For this review, take the finished solid that the model builds, in its own axes (mm). Face numbers are marked on the shaded views. A direction names the side the tool comes from. Coordinates: 2 decimals unless noted, no trailing zeros. Order: outer loops, then holes, each group sorted by start corner. A loop starts at its lowest first (then second) coordinate and runs counter-clockwise, first axis right, second up. Notation, with made-up numbers: (-14.5, 5.5) -> (-9.5, 5.5) arc R22 ccw to (-9.5, 24.5) -> close; hole circle Ø10 at (66.5, 53.5). An arc over 180 degrees is marked (long way). Return JSON: item names as keys, results as strings. Group by question number.
Item 1: Take a section at B-B (y = 1.65). Count the separate pieces of the cut face and the enclosed holes in it, then the cut area to 3 significant figures.
Item 2: Insertion check: pin 1 (1.3 mm diameter, centred on x = 23, y = 3, fed in from +Z); pin 2 (1.8 mm diameter, centred on y = 1.5, z = 110.5, fed in from +X); pin 3 (3 mm diameter, centred on y = 1, z = 70, fed in from -X); pin 4 (2.5 mm diameter, centred on x = 9.43, z = 32.32, fed in from -Y). Each pin has a flat end and moves straight along its axis. Give the tip position at first contact, or say it passes through.
Item 3: For line 1 along X through (y, z) = (2.45, 109); line 2 along X through (y, z) = (1.85, 101); line 3 along X through (y, z) = (3.5, 42), list the stretches that pass through material, from the lowest coordinate up.
Item 4: Machinability: for the marked faces 1 and 2, which of the approach directions +Z, -Z, +X, -X, +Y, -Y give a long, thin tool a straight path to every point of the face, cutting with its end or side? Answer none if there is none.
Item 5: Take a section at C-C (z = 75.5). Write out the cut boundary in (x, y).
Item 6: Take a section at A-A (x = -30). Write out the cut boundary in (y, z).
```python
from build123d import *

# Parameters (mm, degrees)
SKETCH2_R           = 3.0000000000000018
SKETCH2_R_2         = 1.4999999999993736
SKETCH2_R_3         = 1.5000000000000009
SKETCH2_R_4         = 1.4999999999993723
BOSS_EXTRUDE1_DEPTH = 5
FILLET1_R           = 1.5
FILLET3_R           = 10
FILLET5_R           = 10
CHAMFER1_SIZE       = 4.5
FILLET6_R           = 6
FILLET7_R           = 4
FILLET8_R           = 2
FILLET9_R           = 30
CUT_EXTRUDE1_DEPTH  = 142.21634167657882
FILLET10_R          = 1


with BuildPart() as part:
    # Sketch2 → Boss-Extrude1 (new body)
    with BuildSketch(Plane(origin=(0, 0, 0), x_dir=(1, 0, 0), z_dir=(0, 1, 0))):
        with BuildLine():
            Line((-46.189355852298796, -96.42025186017804), (-39.496927389393186, -89.72782339727232))
            Line((-39.496927389393186, -89.72782339727232), (17.913506363615255, -32.31738964426288))
            Line((17.913506363615255, -32.31738964426288), (24.678224989376695, -32.31738964426288))
            Line((24.678224989376695, -32.31738964426288), (24.678224989376428, -17.06738964426295))
            Line((24.678224989376428, -17.06738964426295), (-7.595965049770856, -17.06738964426337))
            Line((-7.595965049770856, -17.06738964426337), (-7.595965049770857, -24.067389644263372))
            Line((-7.595965049770857, -24.067389644263372), (-9.321775010623746, -27.06012368042446))
            Line((-9.321775010623746, -27.06012368042446), (-9.32177501062375, -37.06738964426337))
            Line((-9.32177501062375, -37.06738964426337), (-9.321775010623757, -42.58210827002507))
            Line((-9.321775010623753, -42.58210827002507), (-54.6598701272448, -87.9202033866469))
            Line((-54.6598701272448, -87.9202033866469), (-60.17458875300816, -87.92020338664692))
            ThreePointArc((-60.17458875300816, -87.92020338664692), (-63.00301587775435, -89.09177626190073), (-64.17458875300817, -91.92020338664692))
            Line((-64.17458875300817, -91.92020338664692), (-64.17458875300817, -97.92020338664689))
            Line((-64.17458875300817, -97.92020338664689), (-70.17458875301077, -97.92020338664689))
            ThreePointArc((-70.17458875301077, -97.92020338664689), (-72.6339398041774, -98.76558892412923), (-74.05374095021992, -100.9444071830841))
            Line((-74.05374095021992, -100.9444071830841), (-77.14515150148509, -113.23391188563446))
            Line((-77.14515150148509, -113.23391188563446), (-71.4882972519927, -118.89076613512684))
            Line((-71.4882972519927, -118.89076613512684), (-59.047429208957894, -115.75810794021132))
            ThreePointArc((-59.047429208957894, -115.75810794021132), (-56.9723521770992, -114.3172183869977), (-56.174588753010745, -111.92020338664949))
            Line((-56.174588753010745, -111.92020338664949), (-56.174588753010745, -105.92020338664949))
            Line((-56.174588753010745, -105.92020338664949), (-50.174588753008145, -105.92020338664949))
            ThreePointArc((-50.174588753008145, -105.92020338664949), (-47.34616162826196, -104.74863051139567), (-46.174588753008145, -101.92020338664949))
            Line((-46.174588753008145, -101.92020338664949), (-46.17464642427909, -101.89872393503671))
            Line((-46.17464642427909, -101.89872393503671), (-46.189355852298796, -96.42025186017804))
        make_face()
        Polygon((-70.26446914062754, -114.4577399969996), (-72.71257361922765, -112.00963551839949), (-71.33075600396296, -106.51639746436214), (-66.89210317428027, -106.51639746436214), (-64.77078283072062, -108.63771780792177), (-64.7707828307206, -113.0744087552009), align=None, mode=Mode.SUBTRACT)
        with BuildLine():
            ThreePointArc((-61.67458875301074, -108.42020338664949), (-60.17458875301075, -106.92020338664949), (-58.67458875301077, -108.42020338664949))
            Line((-58.67458875301077, -108.42020338664949), (-58.674588753010774, -111.92020338664949))
            ThreePointArc((-58.674588753010774, -111.92020338664949), (-60.17458875301075, -113.42020338664946), (-61.67458875301073, -111.92020338664949))
            Line((-61.67458875301073, -111.92020338664949), (-61.67458875301074, -108.42020338664949))
        make_face(mode=Mode.SUBTRACT)
        with BuildLine():
            ThreePointArc((-66.67458875301074, -100.42020338664692), (-65.17458875301071, -101.92020338664692), (-66.67458875301074, -103.42020338664692))
            Line((-66.67458875301074, -103.42020338664692), (-70.17458875301077, -103.42020338664692))
            ThreePointArc((-70.17458875301077, -103.42020338664692), (-71.67458875301075, -101.92020338664692), (-70.17458875301077, -100.42020338664692))
            Line((-70.17458875301077, -100.4202033866469), (-66.67458875301074, -100.4202033866469))
        make_face(mode=Mode.SUBTRACT)
        with Locations(Location((-60.174588753008145, -101.92020338664949, 0), (0, 0, 270))):
            Circle(SKETCH2_R, mode=Mode.SUBTRACT)
        with BuildLine():
            ThreePointArc((-53.67458875300815, -103.42020338664949), (-55.17458875300815, -101.92020338664949), (-53.67458875300815, -100.42020338664949))
            Line((-53.67458875300815, -100.42020338664949), (-50.174588753008145, -100.42020338664949))
            ThreePointArc((-50.174588753008145, -100.42020338664949), (-48.67458875300816, -101.92020338664949), (-50.174588753008145, -103.42020338664949))
            Line((-50.174588753008145, -103.42020338664949), (-53.67458875300815, -103.42020338664949))
        make_face(mode=Mode.SUBTRACT)
        with BuildLine():
            ThreePointArc((-58.67458875300815, -95.42020338664692), (-60.17458875300815, -96.9202033866469), (-61.67458875300815, -95.42020338664692))
            Line((-61.674588753008145, -95.42020338664692), (-61.67458875300816, -91.92020338664692))
            ThreePointArc((-61.67458875300816, -91.92020338664692), (-60.174588753008145, -90.42020338664689), (-58.67458875300813, -91.92020338664692))
            Line((-58.67458875300813, -91.92020338664692), (-58.674588753008145, -95.42020338664692))
        make_face(mode=Mode.SUBTRACT)
        with Locations(Location((-1.1783767284213562, -42.92399136206118, 0), (0, 0, 270))):
            Circle(SKETCH2_R_2, mode=Mode.SUBTRACT)
        with Locations(Location((-3.3217750106237407, -28.067389644263372, 0), (0, 0, 270))):
            Circle(SKETCH2_R_3, mode=Mode.SUBTRACT)
        with Locations(Location((9.428224989376764, -32.31738964426288, 0), (0, 0, 270))):
            Circle(SKETCH2_R_4, mode=Mode.SUBTRACT)
        Polygon((1.0820753752795897, -25.575281589539195), (-1.459873180493811, -22.79599601598655), (-1.4598731804937872, -21.06738964426295), (17.849797864630506, -21.06738964426295), (11.740910030340089, -27.17627747855337), (10.272484798754686, -26.22755837455273), align=None, mode=Mode.SUBTRACT)
    extrude(amount=BOSS_EXTRUDE1_DEPTH)

    # Fillet1
    # the kernel refuses this fillet: 1.5 mm, written as the material it adds along each edge
    with BuildSketch(Plane(origin=(1.0820753752795897, 0, 25.575281589539195), x_dir=(0.9974908468725838, 0, 0.07079555357093803), z_dir=(0, 1, 0))) as fillet1_piece_1:
        with BuildLine():
            CenterArc((FILLET1_R * 0.398900109333, FILLET1_R), FILLET1_R, 226.50587582859146, 43.4941241714086)
            Line((-FILLET1_R * 0.289380073746, FILLET1_R * 0.274555040282), (0, 0))
            Line((0, 0), (FILLET1_R * 0.398900109333, 0))
        make_face()
    extrude(amount=5)
    with BuildSketch(Plane(origin=(-1.459873180493811, 0, 22.79599601598655), x_dir=(1.372e-14, 0, -1), z_dir=(0, 1, 0))) as fillet1_piece_2:
        with BuildLine():
            CenterArc((FILLET1_R * 0.388338270451, -FILLET1_R), FILLET1_R, 89.99999999999997, 42.44619337739144)
            Line((-FILLET1_R * 0.286559260205, -FILLET1_R * 0.262088539786), (0, 0))
            Line((0, 0), (FILLET1_R * 0.388338270451, 0))
        make_face()
    extrude(amount=5)
    with BuildSketch(Plane(origin=(-1.459873180493787, 0, 21.06738964426295), x_dir=(1, 0, 0), z_dir=(0, 1, 0))) as fillet1_piece_3:
        with BuildLine():
            CenterArc((FILLET1_R, -FILLET1_R), FILLET1_R, 90, 89.99999999999918)
            Line((-2.087e-14, -FILLET1_R), (0, 0))
            Line((0, 0), (FILLET1_R, 0))
        make_face()
    extrude(amount=5)
    with BuildSketch(Plane(origin=(11.740910030340089, 0, 27.17627747855337), x_dir=(-0.839945220222329, 0, -0.5426711960530642), z_dir=(0, 1, 0))) as fillet1_piece_4:
        with BuildLine():
            CenterArc((FILLET1_R * 0.807844840446, -FILLET1_R), FILLET1_R, 89.99999999999994, 77.86566453571226)
            Line((-FILLET1_R * 0.169812603282, -FILLET1_R * 0.789795521639), (0, 0))
            Line((0, 0), (FILLET1_R * 0.807844840446, -3e-17))
        make_face()
    extrude(amount=5)
    with BuildSketch(Plane(origin=(17.849797864630506, 0, 21.06738964426295), x_dir=(-0.7071067811865475, 0, 0.7071067811865475), z_dir=(0, 1, 0))) as fillet1_piece_5:
        with BuildLine():
            CenterArc((FILLET1_R * 2.41421356237, -FILLET1_R), FILLET1_R, 89.99999999999994, 135.00000000000006)
            Line((FILLET1_R * 1.70710678119, -FILLET1_R * 1.70710678119), (0, 0))
            Line((0, 0), (FILLET1_R * 2.41421356237, 1e-17))
        make_face()
    extrude(amount=5)
    # the kernel refuses this fillet: 1.5 mm, written as the material it takes off along each edge
    with BuildSketch(Plane(origin=(10.27248479875469, -0.9630450228974294, 26.22755837455273), x_dir=(0.8399452202223279, 0, 0.5426711960530661), z_dir=(0, 1, 0))) as fillet1_2_piece_1:
        with BuildLine():
            CenterArc((FILLET1_R * 0.256812006106, -FILLET1_R), FILLET1_R, 90.00000000000006, 28.805982084511456)
            Line((-FILLET1_R * 0.225033157983, -FILLET1_R * 0.123743623222), (0, 0))
            Line((0, 0), (FILLET1_R * 0.256812006106, 2e-17))
        make_face()
    extrude(amount=6.92609004579486, mode=Mode.SUBTRACT)

    # Fillet3
    fillet3_edges = [part.edges().sort_by_distance(p)[0] for p in [
        (17.913506363615255, 2.5, 32.31738964426288),
    ]]
    fillet(fillet3_edges, radius=FILLET3_R)

    # Fillet5
    fillet5_edges = [part.edges().sort_by_distance(p)[0] for p in [
        (-9.321775010623755, 2.5, 42.58210827002507),
    ]]
    fillet(fillet5_edges, radius=FILLET5_R)

    # Chamfer1
    chamfer1_edges = [part.edges().sort_by_distance(p)[0] for p in [
        (-64.17458875300817, 2.5, 97.92020338664689),
        (-56.174588753010745, 2.5, 105.92020338664949),
    ]]
    chamfer(chamfer1_edges, length=CHAMFER1_SIZE)

    # Fillet6
    fillet6_edges = [part.edges().sort_by_distance(p)[0] for p in [
        (-64.17458875300817, 2.5, 93.42020338664689),
        (-68.67458875300817, 2.5, 97.92020338664689),
        (-56.174588753010745, 2.5, 110.42020338664949),
        (-51.674588753010745, 2.5, 105.92020338664949),
    ]]
    fillet(fillet6_edges, radius=FILLET6_R)

    # Fillet7
    fillet7_edges = [part.edges().sort_by_distance(p)[0] for p in [
        (-71.4882972519927, 2.5, 118.89076613512684),
        (-77.14515150148509, 2.5, 113.23391188563446),
    ]]
    fillet(fillet7_edges, radius=FILLET7_R)

    # Fillet8
    fillet8_edges = [part.edges().sort_by_distance(p)[0] for p in [
        (-72.71257361922765, 2.5, 112.00963551839949),
        (-70.26446914062754, 2.5, 114.4577399969996),
        (-64.7707828307206, 2.5, 113.0744087552009),
        (-64.77078283072062, 2.5, 108.63771780792177),
        (-66.89210317428027, 2.5, 106.51639746436214),
        (-71.33075600396296, 2.5, 106.51639746436214),
    ]]
    fillet(fillet8_edges, radius=FILLET8_R)

    # Fillet9
    fillet9_edges = [part.edges().sort_by_distance(p)[0] for p in [
        (-54.6598701272448, 2.5, 87.9202033866469),
        (-46.189355852298796, 2.5, 96.42025186017804),
    ]]
    fillet(fillet9_edges, radius=FILLET9_R)

    # Sketch4 → Cut-Extrude1 (cut, through all)
    with BuildSketch(Plane(origin=(0, 5, 0), x_dir=(1, 0, 0), z_dir=(0, 1, 0))):
        Polygon((-9.321775010623751, -28.81997264629415), (-7.82177501062375, -30.31997264629416), (-7.821775010623751, -34.31997264629416), (-9.321775010623751, -35.819972646294175), align=None)
    extrude(amount=-CUT_EXTRUDE1_DEPTH, mode=Mode.SUBTRACT)

    # Fillet10
    fillet10_edges = [part.edges().sort_by_distance(p)[0] for p in [
        (-7.595965049770856, 2.5, 17.06738964426337),
        (24.678224989376428, 2.5, 17.06738964426295),
        (24.678224989376695, 2.5, 32.31738964426288),
    ]]
    fillet(fillet10_edges, radius=FILLET10_R)


solid = part.part
```
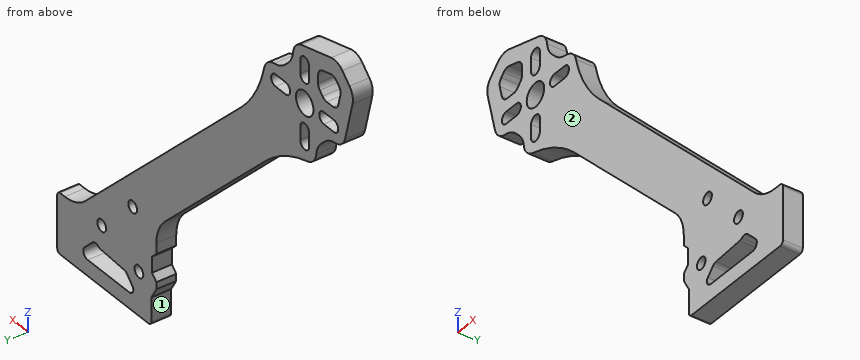
Findings below:
{
 "1": {"separate pieces": "1", "enclosed holes": "10", "area": "1,950 mm2"},
 "2": {"pin 1": "stops at z = 32.32", "pin 2": "stops at x = -55.2", "pin 3": "stops at x = -38.24", "pin 4": "passes through"},
 "3": {"line 1": "x = -76.08 to -71.96, -64.83 to -61.67, -58.67 to -54.74", "line 2": "x = -74.07 to -71.36, -65.49 to -63.03, -57.32 to -54.86, -48.99 to -45.78", "line 3": "x = -9.98 to -2.36, 0 to 8.23"},
 "4": {"face 1": "-Z, -X, +Y, -Y", "face 2": "+Z, -Z, +X, -X, -Y"},
 "5": {"outline": "(-42.24, 0) -> (-25.27, 0) -> (-25.27, 5) -> (-42.24, 5) -> close"},
 "6": {"outline": "(0, 63.26) -> (5, 63.26) -> (5, 80.23) -> (0, 80.23) -> close"}
}
